Verification items for this drawing (mm, ordinates from the low corner). A direction names the side the tool comes from. Give positions to 0.01 mm unless a question says otherwise; leave off trailing zeros. Order: outer loops, then holes, each group sorted by start corner. A loop starts at its lowest first (then second) coordinate and runs counter-clockwise, first axis right, second up. Notation, with made-up numbers: M 45,24 L 54,24 A9 cw 54,37 Z; hole C -11,23 d3. An arc over 180 degrees is marked long. Answer as a JSON object with one key per item and string values.
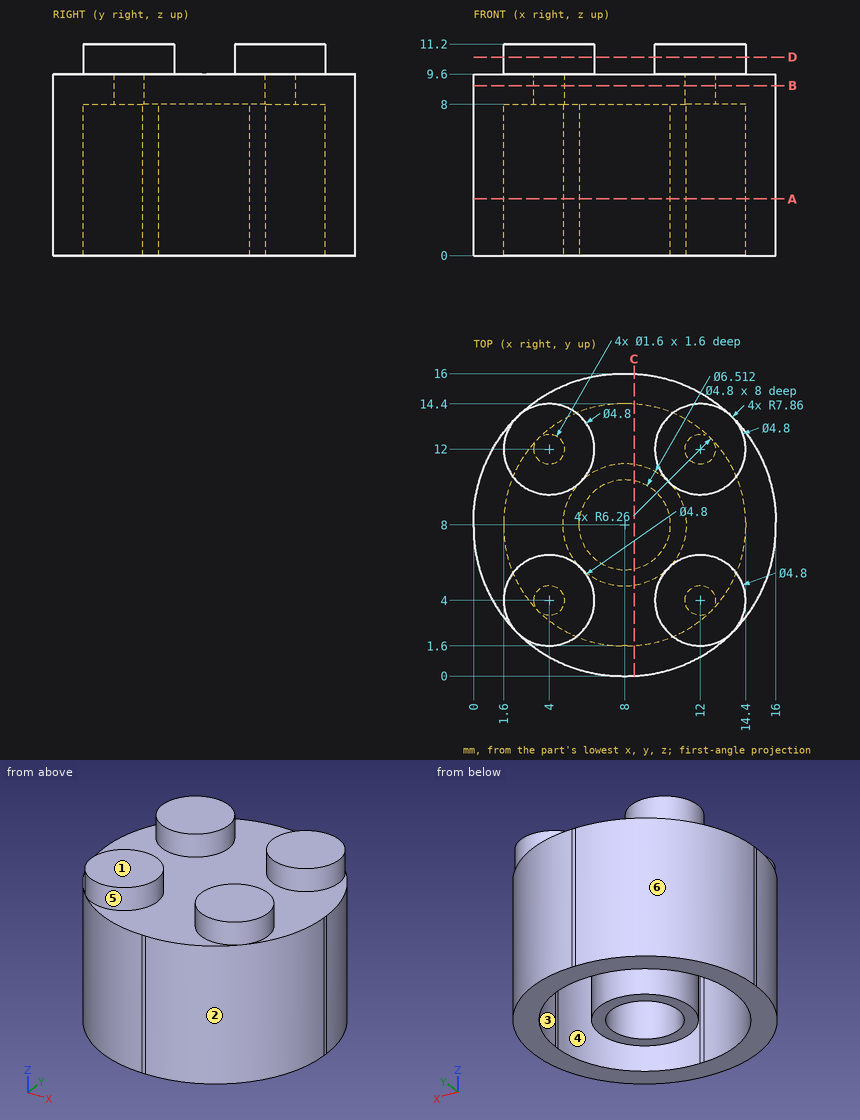
Q1. Gauge pin test, flat ends, axial feed: pin 1 Ø1 at (x, y) = (7, 12.5) entering from +Z; pin 2 Ø1 at (y, z) = (6.5, 4.5) entering from +X; pin 3 Ø2.5 at (x, y) = (9, 8.5) entering from -Z. Record the tip position at first contact, or that the pin passes through.
Resolved:
{"pin 1": "stops at z = 9.6", "pin 2": "stops at x = 15.95", "pin 3": "stops at z = 8"}
Q2. Tool access check on the marked faces 4, 5 and 6. Record the directions out of +Z, -Z, +X, -X, +Y, -Y that give a thin tool (end or side, any length) a straight path to the whole face; none if there is none.
Resolved:
{"face 4": "-Z", "face 5": "+Z", "face 6": "+Z, -Z, -X, +Y"}
Q3. Material ranges on L1, parallel to X at y = 8, z = 2.5; L2, parallel to Y at x = 12, z = 8.55, recorded low to high.
Resolved:
{"L1": "x = 0 to 1.6, 4.74 to 5.6, 10.4 to 11.26, 14.4 to 16", "L2": "y = 1.01 to 3.2, 4.8 to 11.2, 12.8 to 14.99"}
Q4. Section check C-C on x = 8.5. Record the cut outline in (y, z).
Resolved:
{"outline": "M 0.01,0 L 1.61,0 L 1.61,8 L 4.78,8 L 4.78,0 L 5.65,0 L 5.65,8 L 10.35,8 L 10.35,0 L 11.22,0 L 11.22,8 L 14.39,8 L 14.39,0 L 15.99,0 L 15.99,9.6 L 0.01,9.6 Z"}
Q5. Section check A-A on z = 3. Record the cut outline in (x, y), then the cut area to 3 significant figures.
Resolved:
{"outline": "M 0,7.86 A7.86 ccw 7.86,0 L 8.14,0 A7.86 ccw 16,7.86 L 16,8.14 A7.86 ccw 8.14,16 L 7.86,16 A7.86 ccw 0,8.14 Z; C 8,8 d6.51; hole M 1.6,7.86 A6.26 ccw 7.86,1.6 L 8.14,1.6 A6.26 ccw 14.4,7.86 L 14.4,8.14 A6.26 ccw 8.14,14.4 L 7.86,14.4 A6.26 ccw 1.6,8.14 Z; hole C 8,8 d4.8", "area": "88.0 mm²"}
Q6. Release check for a two-part mould opening along Y. For the marked faces 1, 2 and 3 record: +Y half, -Y half, draft (parallel to the pull), parting line (faces both ways), or undercut.
Resolved:
{"face 1": "draft", "face 2": "-Y half", "face 3": "undercut"}
Q7. Section check D-D on z = 10.5. Record the cut outline in (x, y).
Resolved:
{"outline": "C 4,4 d4.8; C 4,12 d4.8; C 12,4 d4.8; C 12,12 d4.8"}
Q8. Section check B-B on z = 9. Record the cut outline in (x, y), then the cut area to 3 significant figures.
Resolved:
{"outline": "M 0,7.86 A7.86 ccw 7.86,0 L 8.14,0 A7.86 ccw 16,7.86 L 16,8.14 A7.86 ccw 8.14,16 L 7.86,16 A7.86 ccw 0,8.14 Z; hole C 4,4 d1.6; hole C 4,12 d1.6; hole C 12,4 d1.6; hole C 12,12 d1.6", "area": "195 mm²"}
